The listing builds one solid part. Answer for the finished solid, in the listing's coordinates (mm). Face numbers are marked on the shaded views. A direction names the side the tool comes from. Give positions to 0.01 mm unless a question says otherwise; leave off trailing zeros. Write each loop counter-clockwise with the first axis right and the second up, starting at its lowest first coordinate (ties: lowest second). Pieces come first, ordered by that corner, then holes. Notation, with made-up numbers: M 87.5,4.5 L 94.5,4.5 A19 cw 94.5,37.5 Z; hole C 69.5,68.25 d3. An arc over 180 degrees is marked long. Return JSON: item names as keys, results as strings.
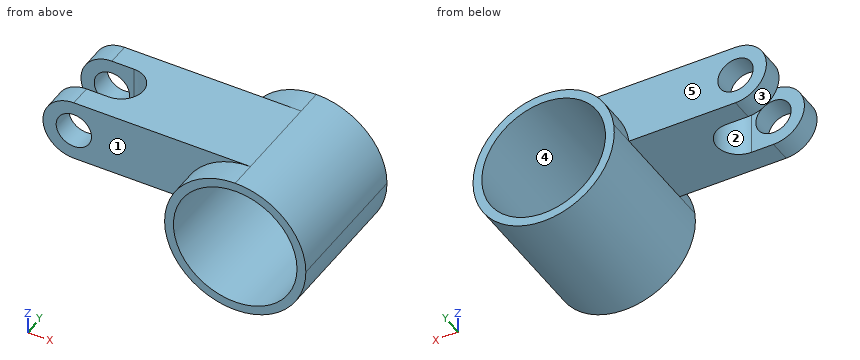
from build123d import *

# Parameters (mm, degrees)
F0_R     = 14
F1_DEPTH = 16
F0_R_2   = 4
F2_DEPTH = 10
F3_W     = 10
F3_H     = 10
F4_DEPTH = 25


with BuildPart() as f1:
    # F0 (on Front) → F1 (new body, symmetric)
    with BuildSketch(Plane.XZ):
        with BuildLine():
            ThreePointArc((7.437397, 2), (22.309938, -15.968596), (39.311905, 0))
            ThreePointArc((39.311905, 0), (34.625613, 11.313708), (23.311905, 16))
            ThreePointArc((23.311905, 16), (12.7289, 12), (7.437397, 2))
        make_face()
        with Locations((23.311905, 0)):
            Circle(F0_R, mode=Mode.SUBTRACT)
    extrude(amount=F1_DEPTH, both=True)

    # F0 (on Front) → F2 (join, symmetric)
    with BuildSketch(Plane.XZ):
        with BuildLine():
            ThreePointArc((7.437397, 2), (12.7289, 12), (23.311905, 16))
            Line((23.311905, 16), (-16.688095, 16))
            ThreePointArc((-16.688095, 16), (-23.688095, 9), (-16.688095, 2))
            Line((-16.688095, 2), (7.437397, 2))
        make_face()
        with Locations((-16.688095, 9)):
            Circle(F0_R_2, mode=Mode.SUBTRACT)
    extrude(amount=F2_DEPTH, both=True)

    # F3 (on face) → F4 (cut)
    with BuildSketch(Plane.XY.offset(16)):
        with Locations((-21.688095, 0)):
            Rectangle(F3_W, F3_H)
        with BuildLine():
            Line((-11.688095, 5), (-16.688095, 5))
            Line((-16.688095, 5), (-16.688095, -5))
            Line((-16.688095, -5), (-11.688095, -5))
            ThreePointArc((-11.688095, -5), (-6.688095, 0), (-11.688095, 5))
        make_face()
    extrude(amount=-F4_DEPTH, mode=Mode.SUBTRACT)


solid = f1.part
Item 1: Find the intervals of material crossed by line 1 (Y direction, x = -18, z = 3); line 2 (X direction, y = -8, z = 9); line 3 (X direction, y = 14, z = -0.5), in increasing order.
Geometry results:
{"line 1": "y = -10 to -5, 5 to 10", "line 2": "x = -23.69 to -20.69, -12.69 to 12.59, 34.04 to 36.54", "line 3": "x = 7.32 to 9.32, 37.3 to 39.3"}
Item 2: A cutting plane is placed at C-C, the plane y = -6.5. Write down the section's boundary in (x, z), plus the area to 3 significant figures.
Geometry results:
{"outline": "M -16.69,2 L 7.44,2 A16 ccw long 39.31,0 A16 ccw 23.31,16 L -16.69,16 A7 ccw Z; hole C -16.69,9 d8; hole C 23.31,0 d28", "area": "606 mm2"}
Item 3: A cutting plane is placed at D-D, the plane z = -1.5. Write down the section's boundary in (x, y).
Geometry results:
{"outline": "M 7.38,-16 L 9.39,-16 L 9.39,16 L 7.38,16 Z; M 37.23,-16 L 39.24,-16 L 39.24,16 L 37.23,16 Z"}
Item 4: Which of the six approach directions +Z, -Z, +X, -X, +Y, -Y give full straight-line access (tool end or side, diameter ignored) to the marked faces 1 and 2?
Geometry results:
{"face 1": "+Z, -X, -Y", "face 2": "+Z, -Z, -X"}
Item 5: Determine the mould class of the marked faces 3, 4 and 5 for opening direction Z: +Z half, -Z half, draft (parallel to the pull), parting line (faces both ways), or undercut.
Geometry results:
{"face 3": "parting line", "face 4": "undercut", "face 5": "draft"}
Item 6: A cutting plane is placed at B-B, the plane x = 21. Write down the section's boundary in (y, z), plus the area to 3 significant figures.
Geometry results:
{"outline": "M -16,-15.83 L 16,-15.83 L 16,-13.81 L -16,-13.81 Z; M -16,13.81 L 16,13.81 L 16,15.83 L 10,15.83 L 10,16 L -10,16 L -10,15.83 L -16,15.83 Z", "area": "133 mm2"}
Item 7: A cutting plane is placed at A-A, the plane z = 9. Write down the section's boundary in (x, y), plus the area to 3 significant figures.
Geometry results:
{"outline": "M -23.69,-10 L -20.69,-10 L -20.69,-5 L -23.69,-5 Z; M -23.69,5 L -20.69,5 L -20.69,10 L -23.69,10 Z; M -12.69,-10 L 10.08,-10 L 10.08,-16 L 12.59,-16 L 12.59,16 L 10.08,16 L 10.08,10 L -12.69,10 L -12.69,5 L -11.69,5 A5 cw -11.69,-5 L -12.69,-5 Z; M 34.04,-16 L 36.54,-16 L 36.54,16 L 34.04,16 Z", "area": "596 mm2"}
Item 8: Given pin 1 Ø4 at (x, z) = (-9, 10.5) entering from -Y; pin 2 Ø6.5 at (x, z) = (-16.69, 9) entering from -Y; pin 3 Ø4 at (x, z) = (-10.5, 7.5) entering from +Y; pin 4 Ø10 at (y, z) = (4, 2.5) entering from -X, each flat-ended and moving along its own axis, determine where each tip first touches the part or whether it passes through.
Geometry results:
{"pin 1": "stops at y = -10", "pin 2": "passes through", "pin 3": "stops at y = 10", "pin 4": "stops at x = -23.5"}
